from build123d import *

# Parameters (mm, degrees)
SKETCH1_W         = 102
SKETCH1_H         = 56
SKETCH1_W_2       = 61
SKETCH1_H_2       = 45
FRONT_DEPTH       = 2
SKETCH2_W         = 99.6
SKETCH2_H         = 53.6
SKETCH2_W_2       = 97.2
SKETCH2_H_2       = 51.2
WALLS_DEPTH       = 2
SKETCH3_R         = 1.45
SCREW_SPOTS_DEPTH = 7


with BuildPart() as part:
    # Sketch1 → Front (new body)
    with BuildSketch(Plane.XY):
        Rectangle(SKETCH1_W, SKETCH1_H)
        Rectangle(SKETCH1_W_2, SKETCH1_H_2, mode=Mode.SUBTRACT)
    extrude(amount=FRONT_DEPTH)

    # Sketch2 → WALLS (add)
    with BuildSketch(Plane(origin=(0, 0, 0), x_dir=(-1, 0, 0), z_dir=(0, 0, -1))):
        Rectangle(SKETCH2_W, SKETCH2_H)
        Rectangle(SKETCH2_W_2, SKETCH2_H_2, mode=Mode.SUBTRACT)
    extrude(amount=WALLS_DEPTH)

    # Sketch3 → SCREW_SPOTS (add)
    with BuildSketch(Plane(origin=(0, 0, 0), x_dir=(-1, 0, 0), z_dir=(0, 0, -1))):
        with Locations((-41, 21.9)):
            Circle(SKETCH3_R)
        with Locations((35.3, 21.9)):
            Circle(SKETCH3_R)
        with Locations((-41, -22.2)):
            Circle(SKETCH3_R)
        with Locations((35.3, -22.2)):
            Circle(SKETCH3_R)
    extrude(amount=SCREW_SPOTS_DEPTH)


solid = part.part
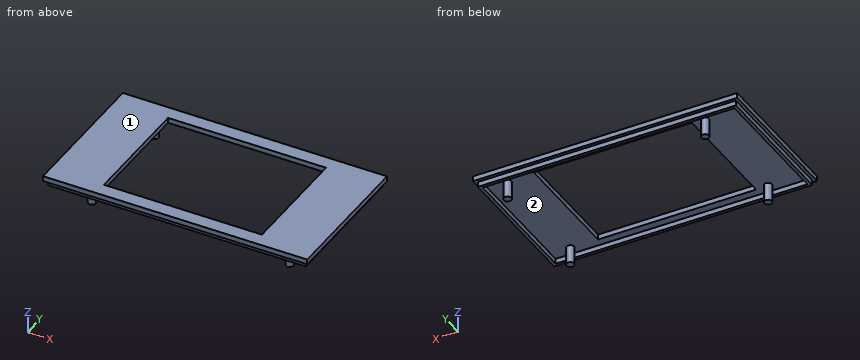
Source: CAD feature listing. Evaluate the final solid. Frame: model axes, mm. Face numbers are marked on the shaded views. Coordinates: 2 decimals unless noted, no trailing zeros. Loops run counter-clockwise (first coordinate to the right, second up) from the corner with the lowest first, then second, coordinate; pieces in that order, holes last. Notation, with made-up numbers: M 42.25,52.5 L 48.25,52.5 A22 cw 48.25,78.5 Z; hole C 36.5,-10 d10. An arc over 180 degrees is marked long. Answer in a Markdown table with one row per item.
Q1. Draft query along Y for the marked faces 1 and 2. Return one class per face: pulls with the +Y half, pulls with the -Y half, needs draft (parallel to the pull), parting line crosses it, or undercut.
Answers below:
| item | result |
|---|---|
| face 1 | needs draft |
| face 2 | undercut |
Q2. Section B-B on y = 6. Return the cut outline in (x, z), plus the area to 3 significant figures.
Answers below:
| item | result |
|---|---|
| outline | M -51,0 L -49.8,0 L -49.8,-2 L -48.6,-2 L -48.6,0 L -30.5,0 L -30.5,2 L -51,2 Z; M 30.5,0 L 48.6,0 L 48.6,-2 L 49.8,-2 L 49.8,0 L 51,0 L 51,2 L 30.5,2 Z |
| area | 86.8 mm^2 |
Q3. Section A-A on x = -23.5. Return the cut outline in (y, z).
Answers below:
| item | result |
|---|---|
| outline | M -28,0 L -26.8,0 L -26.8,-2 L -25.6,-2 L -25.6,0 L -22.5,0 L -22.5,2 L -28,2 Z; M 22.5,0 L 25.6,0 L 25.6,-2 L 26.8,-2 L 26.8,0 L 28,0 L 28,2 L 22.5,2 Z |
Q4. Section C-C on x = -35.3. Return the cut outline in (y, z).
Answers below:
| item | result |
|---|---|
| outline | M -28,0 L -26.8,0 L -26.8,-2 L -25.6,-2 L -25.6,0 L -23.65,0 L -23.65,-7 L -20.75,-7 L -20.75,0 L 20.45,0 L 20.45,-7 L 23.35,-7 L 23.35,0 L 25.6,0 L 25.6,-2 L 26.8,-2 L 26.8,0 L 28,0 L 28,2 L -28,2 Z |
Q5. First-contact query: pin 1 (0.6 mm diameter, centred on x = -10.5, z = -1.5, fed in from -Y); pin 2 (1 mm diameter, centred on y = 11, z = -1, fed in from +X); pin 3 (1.6 mm diameter, centred on y = 5, z = -1, fed in from -X). Flat tips, straight axial feed; report the tip coordinate or a pass-through.
Answers below:
| item | result |
|---|---|
| pin 1 | stops at y = -26.8 |
| pin 2 | stops at x = 49.8 |
| pin 3 | stops at x = -49.8 |
Q6. Section D-D on z = -3.75. Return the cut outline in (x, y), plus the area to 3 significant figures.
Answers below:
| item | result |
|---|---|
| outline | C -35.3,-22.2 d2.9; C -35.3,21.9 d2.9; C 41,-22.2 d2.9; C 41,21.9 d2.9 |
| area | 26.4 mm^2 |
Q7. Ray query, probe 1 along X at (y, z) = (17.5, -0.75); probe 2 along Y at (x, z) = (28, 1); probe 3 along Y at (x, z) = (4.5, -1). Return the intervals inside material, ascending. Write a range as from..to.
Answers below:
| item | result |
|---|---|
| probe 1 | x = -49.8..-48.6, 48.6..49.8 |
| probe 2 | y = -28..-22.5, 22.5..28 |
| probe 3 | y = -26.8..-25.6, 25.6..26.8 |
